Can you work these out from the model? Positions are in its coordinate system, mm. Face numbers are marked on the shaded views. A direction names the side the tool comes from. Round coordinates to 2 decimals unless told otherwise and drop trailing zeros. Loops run counter-clockwise (first coordinate to the right, second up) from the corner with the lowest first, then second, coordinate; pieces in that order, holes last. Notation, with made-up numbers: (58, 16.5) -> (92, 16.5) arc R19 cw to (92, 50.5) -> close; hole circle Ø4 at (33, 60). An arc over 180 degrees is marked (long way). Answer as a JSON object with one key per item and string values.
```python
from build123d import *
from OCP.BRepFilletAPI import BRepFilletAPI_MakeChamfer

# Parameters (mm, degrees)
BOSS_EXTRUDE1_DEPTH = 16
SKETCH2_R           = 1.4
CUT_EXTRUDE1_DEPTH  = 10
SKETCH3_R           = 1.5
BOSS_EXTRUDE2_DEPTH = 6
CHAMFER1_SIZE       = 0.5
CHAMFER1_SIZE2      = 0.288675135
CHAMFER2_SIZE       = 0.2


with BuildPart() as part:
    # Sketch1 → Boss-Extrude1 (new body)
    with BuildSketch(Plane(origin=(0, 0, 0), x_dir=(1, 0, 0), z_dir=(0, 1, 0))):
        Polygon((1.497494138, 2.800150824), (-1.676254679, 2.696943378), (-3.173748817, -0.103207446), (-1.497494138, -2.800150824), (1.676254679, -2.696943378), (3.173748817, 0.103207446), align=None)
    extrude(amount=BOSS_EXTRUDE1_DEPTH)

    # Sketch2 → Cut-Extrude1 (cut)
    with BuildSketch(Plane(origin=(0, 16, 0), x_dir=(1, 0, 0), z_dir=(0, 1, 0))):
        with Locations(Location((0, 0, 0), (0, 0, 270))):
            Circle(SKETCH2_R)
    extrude(amount=-CUT_EXTRUDE1_DEPTH, mode=Mode.SUBTRACT)

    # Sketch3 → Boss-Extrude2 (add)
    with BuildSketch(Plane.XZ):
        with Locations(Location((0, 0, 0), (0, 0, 270))):
            Circle(SKETCH3_R)
    extrude(amount=BOSS_EXTRUDE2_DEPTH)

    # Chamfer1: one chamfer whose edges measure the first distance from different faces: ONE call of the kernel's chamfer builder (chamfer() names one face for all edges)
    chamfer1_edges_1 = [part.edges().sort_by_distance(p)[0] for p in [
        (0, 16, -1.4),
    ]]
    chamfer1_side_1 = [part.faces().sort_by_distance(p)[0] for p in [
        (0, 11, -1.4),
    ]]
    chamfer1_edges_2 = [part.edges().sort_by_distance(p)[0] for p in [
        (0, -6, 1.5),
    ]]
    chamfer1_side_2 = [part.faces().sort_by_distance(p)[0] for p in [
        (0, -3, 1.5),
    ]]
    chamfer1 = BRepFilletAPI_MakeChamfer(part.part.solid().wrapped)
    for e in chamfer1_edges_1:
        chamfer1.Add(CHAMFER1_SIZE, CHAMFER1_SIZE2, e.wrapped, chamfer1_side_1[0].wrapped)  # the first distance lies on this face
    for e in chamfer1_edges_2:
        chamfer1.Add(CHAMFER1_SIZE, CHAMFER1_SIZE2, e.wrapped, chamfer1_side_2[0].wrapped)  # the first distance lies on this face
    add(Compound.cast(chamfer1.Shape()), mode=Mode.REPLACE)

    # Chamfer2
    chamfer2_edges = [part.edges().sort_by_distance(p)[0] for p in [
        (-2.425001748, 16, -1.296867966),
        (-2.335621478, 16, 1.451679135),
        (0.08938027, 16, 2.748547101),
        (2.425001748, 16, 1.296867966),
        (2.335621478, 16, -1.451679135),
        (-0.08938027, 16, -2.748547101),
    ]]
    chamfer(chamfer2_edges, length=CHAMFER2_SIZE)


solid = part.part
```
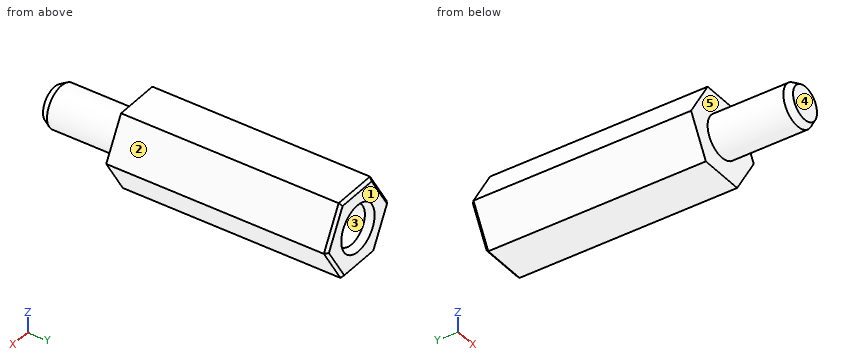
Q1. I want a section at C-C, the plane x = 0. Write out the boundary of the cut face in (y, z), then the cut area to 3 significant figures.
Determined:
{"outline": "(-6, -1.21) -> (-5.5, -1.5) -> (0, -1.5) -> (0, -2.75) -> (15.8, -2.75) -> (16, -2.55) -> (16, -1.69) -> (15.5, -1.4) -> (6, -1.4) -> (6, 1.4) -> (15.5, 1.4) -> (16, 1.69) -> (16, 2.55) -> (15.8, 2.75) -> (0, 2.75) -> (0, 1.5) -> (-5.5, 1.5) -> (-6, 1.21) -> close", "area": "77.7 mm²"}
Q2. I want a section at A-A, the plane y = 14. Write out the boundary of the cut face in (x, z).
Determined:
{"outline": "(-3.17, 0.1) -> (-1.68, -2.7) -> (1.5, -2.8) -> (3.17, -0.1) -> (1.68, 2.7) -> (-1.5, 2.8) -> close; hole circle Ø2.8 at (0, 0)"}
Q3. We'd pull the mould along X, two halves only. Please class the marked faces 1, 2 and 3: pulls with the +X half, pulls with the -X half, needs draft (parallel to the pull), parting line crosses it, or undercut.
Determined:
{"face 1": "needs draft", "face 2": "pulls with the +X half", "face 3": "undercut"}
Q4. I'm going to push flat-ended pins straight in: pin 1 (1 mm diameter, centred on x = -2, y = 11.5, fed in from -Z); pin 2 (2.5 mm diameter, centred on x = 0, z = 0, fed in from +Y); pin 3 (3 mm diameter, centred on y = -3, z = -1.5, fed in from +X); pin 4 (3 mm diameter, centred on x = -1, z = 1, fed in from -Y). Where does each tip first touch, or does it pass through?
Determined:
{"pin 1": "z = -2.7", "pin 2": "y = 6", "pin 3": "x = 1.5", "pin 4": "y = -6"}
Q5. I want a section at D-D, the plane z = -1.95. Write out the boundary of the cut face in (x, y), then the cut area to 3 significant figures.
Determined:
{"outline": "(-2.08, 0) -> (2.03, 0) -> (2.03, 15.8) -> (1.79, 16) -> (-1.85, 16) -> (-2.08, 15.8) -> close", "area": "65.6 mm²"}
Q6. I want a section at B-B, the plane y = 4.5. Write out the boundary of the cut face in (x, z).
Determined:
{"outline": "(-3.17, 0.1) -> (-1.68, -2.7) -> (1.5, -2.8) -> (3.17, -0.1) -> (1.68, 2.7) -> (-1.5, 2.8) -> close"}
Q7. On a 3-axis mill with a long thin cutter (end or side, diameter ignored), from which of +Z, -Z, +X, -X, +Y, -Y can I reach the whole of each face in a straight line? I mean the marked faces 4 and 5. Say none if no direction works.
Determined:
{"face 4": "+Z, -Z, +X, -X, -Y", "face 5": "-Y"}
Q8. If I drill on L1, parallel to Y at x = 1.5, z = 1.7; L2, parallel to X at y = 11.75, z = 0; L3, parallel to Y at x = 0.25, z = 0.85, over which ranges is the centre line in solid material (lowest first)? Write a range as [from, to].
Determined:
{"L1": "[0, 16]", "L2": "[-3.12, -1.4], [1.4, 3.12]", "L3": "[-6, 6]"}
